Check sheet for the modelled part. Datum: model origin and axes. Units: mm. A direction names the side the tool comes from. Round coordinates to 2 decimals unless told otherwise and drop trailing zeros. Loops run counter-clockwise (first coordinate to the right, second up) from the corner with the lowest first, then second, coordinate; pieces in that order, holes last. Notation, with made-up numbers: (-5, -7) - (7, -7) arc R21 ccw to (7, 22) - close; hole circle Ø1 at (-34, 82). An arc over 180 degrees is marked (long way). Put each result on its own line as item: value. Start each with the question number.
Item 1: Section check A-A, the plane z = -24. Record the cut outline in (x, y), and give its area (3 significant figures).
Item 2: Material ranges on line 1 along Y through (x, z) = (-3.25, 218); line 2 along Y through (x, z) = (-1.75, 19); line 3 along Z through (x, y) = (4.75, 4.25), recorded low to high.
Item 3: Gauge pin test, flat ends, axial feed: pin 1 Ø1 at (y, z) = (-4.5, 109.5) entering from -X; pin 2 Ø6 at (x, z) = (-4.5, 142) entering from -Y; pin 3 Ø3 at (x, z) = (3.5, -7) entering from -Y. Record the tip position at first contact, or that the pin passes through.
Item 4: Tool access check on faces 1 (the flat face through (0, 0, 330.2)), 2 (the cylindrical face through (1.38, -6.2, 326.29)), 3 (the cylindrical face through (1.38, -6.2, -326.29)). Record the directions out of +Z, -Z, +X, -X, +Y, -Y that give a thin tool (end or side, any length) a straight path to the whole face; none if there is none.
from build123d import *

# Parameters (mm, degrees)
BOSS_EXTRUDE1_DEPTH     = 330.2
SKETCH2_R               = 8.89
SKETCH2_R_2             = 6.35
CUT_EXTRUDE_THIN1_DEPTH = 7.9375


with BuildPart() as part:
    # Sketch1 → Boss-Extrude1 (new, symmetric)
    with BuildSketch(Plane.XY):
        Polygon((0, 7.332348419), (-6.35, 3.666174209), (-6.35, -3.666174209), (0, -7.332348419), (6.35, -3.666174209), (6.35, 3.666174209), align=None)
    extrude(amount=BOSS_EXTRUDE1_DEPTH, both=True)

    # Sketch2 → Cut-Extrude-Thin1 (cut)
    with BuildSketch(Plane(origin=(0, 0, -330.2), x_dir=(-1, 0, 0), z_dir=(0, 0, -1))):
        Circle(SKETCH2_R)
        Circle(SKETCH2_R_2, mode=Mode.SUBTRACT)
    cut_extrude_thin1 = extrude(amount=-CUT_EXTRUDE_THIN1_DEPTH, mode=Mode.SUBTRACT)

    # Mirror1: Cut-Extrude-Thin1 across plane
    add(cut_extrude_thin1.mirror(Plane.XY), mode=Mode.SUBTRACT)


solid = part.part
Check result:
1. outline: (-6.35, -3.67) - (0, -7.33) - (6.35, -3.67) - (6.35, 3.67) - (0, 7.33) - (-6.35, 3.67) - close
1. area: 140 mm²
2. line 1: -5.46 to 5.46
2. line 2: -6.32 to 6.32
2. line 3: -322.26 to 322.26
3. pin 1: x = -5.77
3. pin 2: y = -6.47
3. pin 3: y = -6.18
4. face 1: +Z, +X, -X, +Y, -Y
4. face 2: +Z
4. face 3: -Z
